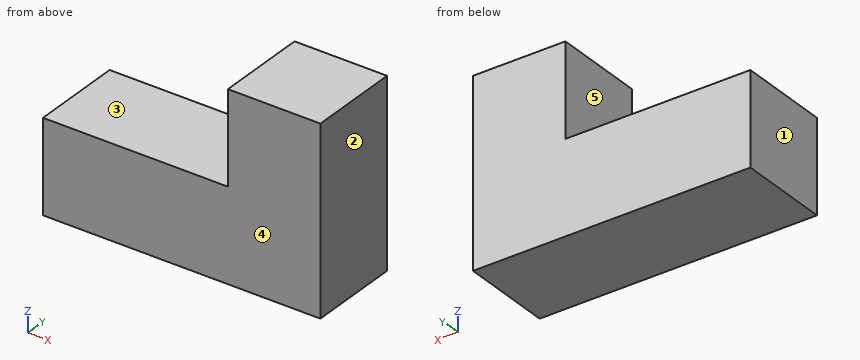
```python
from build123d import *

# Parameters (mm, degrees)
F0_W     = 19.05
F0_H     = 19.05
F1_DEPTH = 19.05


with BuildPart() as f1:
    # F0 (on Front) → F1 (new body)
    with BuildSketch(Plane.XZ):
        Rectangle(F0_W, F0_H)
        with Locations((19.05, 0)):
            Rectangle(F0_W, F0_H)
        with Locations((19.05, 19.05)):
            Rectangle(F0_W, F0_H)
        with Locations((-19.05, 0)):
            Rectangle(F0_W, F0_H)
    extrude(amount=F1_DEPTH)


solid = f1.part
```
Verification items for the finished model (mm, model axes). Face numbers are marked on the shaded views. A direction names the side the tool comes from. Round coordinates to 2 decimals unless told otherwise and drop trailing zeros. Write each loop counter-clockwise with the first axis right and the second up, starting at its lowest first coordinate (ties: lowest second). Pieces come first, ordered by that corner, then holes.
1. Scan lines: L1, parallel to Z at x = -16.5, y = -15 (3 decimals); L2, parallel to X at y = -11, z = 20.5 (3 decimals). Record each from-to range of solid material in increasing order.
2. Section check C-C on x = -15.5. Enter the section's corners in (y, z) (3 decimals).
3. Section check A-A on y = -11. Enter the section's corners in (x, z) (3 decimals).
4. Draft check along X on the marked faces 1, 2 and 3. Enter one of: +X half, -X half, draft (parallel to the pull), parting line (faces both ways), or undercut.
5. Gauge pin test, flat ends, axial feed: P1, Ø4, axis at y = -12, z = 23.5, coming from the -X side (3 decimals); P2, Ø6, axis at x = -12, y = -7.5, coming from the +Z side (3 decimals). Record the tip position at first contact, or that the pin passes through.
6. Section check B-B on z = 25.5. Enter the section's corners in (x, y) (3 decimals).
7. Access from +Z, -Z, +X, -X, +Y, -Y to the whole of each face (thin tool, end or side, straight path). Record for the marked faces 4 and 5.
Answer:
1. L1: z = -9.525 to 9.525
1. L2: x = 9.525 to 28.575
2. outline: (-19.05, -9.525) - (0, -9.525) - (0, 9.525) - (-19.05, 9.525) - close
3. outline: (-28.575, -9.525) - (28.575, -9.525) - (28.575, 28.575) - (9.525, 28.575) - (9.525, 9.525) - (-28.575, 9.525) - close
4. face 1: -X half
4. face 2: +X half
4. face 3: draft
5. P1: stops at x = 9.525
5. P2: stops at z = 9.525
6. outline: (9.525, -19.05) - (28.575, -19.05) - (28.575, 0) - (9.525, 0) - close
7. face 4: +Z, -Z, +X, -X, -Y
7. face 5: +Z, -X, +Y, -Y
